```python
from build123d import *

# Parameters (mm, degrees)
SKETCH1_W           = 121.92
SKETCH1_H           = 63.5
BOSS_EXTRUDE1_DEPTH = 5.08
FILLET1_R           = 7.62
SKETCH2_W           = 9.906
SKETCH2_H           = 9.906
BOSS_EXTRUDE2_DEPTH = 22.86
CUT_EXTRUDE2_REACH  = 142.276
SKETCH5_R           = 10.9982
CUT_EXTRUDE3_REACH  = 142.276
SKETCH6_R           = 1.9939
SKETCH7_R           = 5.08
CUT_EXTRUDE4_DEPTH  = 3.81
SKETCH8_R           = 15.24
CUT_EXTRUDE5_DEPTH  = 2.54
CUT_EXTRUDE6_REACH  = 142.276
SKETCH9_R           = 2.159
CUT_EXTRUDE7_REACH  = 142.276
SKETCH11_W          = 143.390320112
SKETCH11_H          = 95.839563071
CUT_EXTRUDE8_DEPTH  = 5.08
SKETCH14_W          = 9.906
SKETCH14_H          = 9.906
BOSS_EXTRUDE4_DEPTH = 7.62
FILLET2_R           = 4.826
FILLET3_R           = 5.08
SKETCH15_R          = 1.27
CUT_EXTRUDE10_DEPTH = 20.32
CUT_EXTRUDE11_REACH = 142.804
SKETCH16_R          = 2.413
CUT_EXTRUDE12_START = -2.54
SKETCH17_W          = 6.096
SKETCH17_H          = 25.146
SKETCH17_W_2        = 2.38136189
SKETCH17_H_2        = 4.064
CUT_EXTRUDE12_DEPTH = 2.54
CUT_EXTRUDE13_REACH = 142.804


with BuildPart() as part:
    # Sketch1 → Boss-Extrude1 (new body)
    with BuildSketch(Plane(origin=(0, 0, 0), x_dir=(1, 0, 0), z_dir=(0, 1, 0))):
        with Locations((60.96, 31.75)):
            Rectangle(SKETCH1_W, SKETCH1_H)
    extrude(amount=BOSS_EXTRUDE1_DEPTH)

    # Fillet1
    fillet1_edges = [part.edges().sort_by_distance(p)[0] for p in [
        (0, 2.54, -63.5),
        (121.92, 2.54, -63.5),
        (121.92, 2.54, 0),
        (0, 2.54, 0),
    ]]
    fillet(fillet1_edges, radius=FILLET1_R)

    # Sketch2 → Boss-Extrude2 (add)
    with BuildSketch(Plane(origin=(0, 5.08, 0), x_dir=(1, 0, 0), z_dir=(0, 1, 0))):
        with Locations((7.747, 55.753)):
            Rectangle(SKETCH2_W, SKETCH2_H)
        with Locations((114.173, 55.753)):
            Rectangle(SKETCH2_W, SKETCH2_H)
        with Locations((114.173, 7.747)):
            Rectangle(SKETCH2_W, SKETCH2_H)
        with Locations((7.747, 7.747)):
            Rectangle(SKETCH2_W, SKETCH2_H)
    extrude(amount=BOSS_EXTRUDE2_DEPTH)

    # Sketch5 → Cut-Extrude2 (cut, up to next)
    with BuildSketch(Plane.XZ, mode=Mode.PRIVATE) as cut_extrude2_sk1:
        with Locations(Location((49.276, -31.75, 0), (0, 0, 270))):
            Circle(SKETCH5_R)
    cut_extrude2_tool1 = extrude(cut_extrude2_sk1.sketch, amount=-CUT_EXTRUDE2_REACH, mode=Mode.PRIVATE) & part.part
    add(cut_extrude2_tool1.solids().sort_by_distance((49.276, 0, -31.75))[0], mode=Mode.SUBTRACT)

    # Sketch6 → Cut-Extrude3 (cut, up to next)
    with BuildSketch(Plane.XZ, mode=Mode.PRIVATE) as cut_extrude3_sk1:
        with Locations(Location((25.4, -16.51, 0), (0, 0, 270))):
            Circle(SKETCH6_R)
    cut_extrude3_tool1 = extrude(cut_extrude3_sk1.sketch, amount=-CUT_EXTRUDE3_REACH, mode=Mode.PRIVATE) & part.part
    # Sketch6 → Cut-Extrude3 (cut, up to next)
    with BuildSketch(Plane.XZ, mode=Mode.PRIVATE) as cut_extrude3_sk2:
        with Locations(Location((25.4, -46.99, 0), (0, 0, 270))):
            Circle(SKETCH6_R)
    cut_extrude3_tool2 = extrude(cut_extrude3_sk2.sketch, amount=-CUT_EXTRUDE3_REACH, mode=Mode.PRIVATE) & part.part
    add(cut_extrude3_tool1.solids().sort_by_distance((25.4, 0, -16.51))[0], mode=Mode.SUBTRACT)
    add(cut_extrude3_tool2.solids().sort_by_distance((25.4, 0, -46.99))[0], mode=Mode.SUBTRACT)

    # Sketch7 → Cut-Extrude4 (cut)
    with BuildSketch(Plane(origin=(0, 5.08, 0), x_dir=(1, 0, 0), z_dir=(0, 1, 0))):
        with Locations(Location((25.4, 46.99, 0), (0, 0, 270))):
            Circle(SKETCH7_R)
        with Locations(Location((25.4, 16.51, 0), (0, 0, 270))):
            Circle(SKETCH7_R)
    extrude(amount=-CUT_EXTRUDE4_DEPTH, mode=Mode.SUBTRACT)

    # Sketch8 → Cut-Extrude5 (cut)
    with BuildSketch(Plane(origin=(0, 5.08, 0), x_dir=(1, 0, 0), z_dir=(0, 1, 0))):
        with Locations(Location((49.276, 31.75, 0), (0, 0, 270))):
            Circle(SKETCH8_R)
    extrude(amount=-CUT_EXTRUDE5_DEPTH, mode=Mode.SUBTRACT)

    # Sketch9 → Cut-Extrude6 (cut, up to next)
    with BuildSketch(Plane.XZ, mode=Mode.PRIVATE) as cut_extrude6_sk1:
        with Locations(Location((25.4, -16.51, 0), (0, 0, 270))):
            Circle(SKETCH9_R)
    cut_extrude6_tool1 = extrude(cut_extrude6_sk1.sketch, amount=-CUT_EXTRUDE6_REACH, mode=Mode.PRIVATE) & part.part
    # Sketch9 → Cut-Extrude6 (cut, up to next)
    with BuildSketch(Plane.XZ, mode=Mode.PRIVATE) as cut_extrude6_sk2:
        with Locations(Location((25.4, -46.99, 0), (0, 0, 270))):
            Circle(SKETCH9_R)
    cut_extrude6_tool2 = extrude(cut_extrude6_sk2.sketch, amount=-CUT_EXTRUDE6_REACH, mode=Mode.PRIVATE) & part.part
    add(cut_extrude6_tool1.solids().sort_by_distance((25.4, 0, -16.51))[0], mode=Mode.SUBTRACT)
    add(cut_extrude6_tool2.solids().sort_by_distance((25.4, 0, -46.99))[0], mode=Mode.SUBTRACT)

    # Sketch10 → Cut-Extrude7 (cut, up to next)
    with BuildSketch(Plane.XZ, mode=Mode.PRIVATE) as cut_extrude7_sk1:
        with BuildLine():
            Line((52.324, -42.502333328), (52.324, -43.561))
            Line((52.324, -43.561), (46.228, -43.561))
            Line((46.228, -43.561), (46.228, -42.502333328))
            ThreePointArc((46.228, -42.502333328), (40.758626429, -38.985836057), (38.172393559, -33.02))
            Line((38.172393559, -33.02), (36.957, -33.02))
            Line((36.957, -33.02), (36.957, -30.48))
            Line((36.957, -30.48), (38.172393559, -30.48))
            ThreePointArc((38.172393559, -30.48), (40.758626429, -24.514163943), (46.228, -20.997666672))
            Line((46.228, -20.997666672), (46.228, -19.939))
            Line((46.228, -19.939), (52.324, -19.939))
            Line((52.324, -19.939), (52.324, -20.997666672))
            ThreePointArc((52.324, -20.997666672), (60.452, -31.75), (52.324, -42.502333328))
        make_face()
    cut_extrude7_tool1 = extrude(cut_extrude7_sk1.sketch, amount=-CUT_EXTRUDE7_REACH, mode=Mode.PRIVATE) & part.part
    add(cut_extrude7_tool1.solids().sort_by_distance((49.190062, 0, -31.75))[0], mode=Mode.SUBTRACT)

    # Sketch11 → Cut-Extrude8 (cut)
    with BuildSketch(Plane(origin=(0, 27.94, 0), x_dir=(1, 0, 0), z_dir=(0, 1, 0))):
        with Locations((59.888985007, 35.781035454)):
            Rectangle(SKETCH11_W, SKETCH11_H)
    extrude(amount=-CUT_EXTRUDE8_DEPTH, mode=Mode.SUBTRACT)

    # Sketch14 → Boss-Extrude4 (add)
    with BuildSketch(Plane(origin=(0, 22.86, 0), x_dir=(1, 0, 0), z_dir=(0, 1, 0))):
        with Locations((114.173, 7.747)):
            Rectangle(SKETCH14_W, SKETCH14_H)
        with Locations((7.747, 7.747)):
            Rectangle(SKETCH14_W, SKETCH14_H)
        with Locations((114.173, 55.753)):
            Rectangle(SKETCH14_W, SKETCH14_H)
        with Locations((7.747, 55.753)):
            Rectangle(SKETCH14_W, SKETCH14_H)
    extrude(amount=BOSS_EXTRUDE4_DEPTH)

    # Fillet2
    fillet2_edges = [part.edges().sort_by_distance(p)[0] for p in [
        (2.794, 17.78, -2.794),
        (119.126, 17.78, -2.794),
        (119.126, 17.78, -60.706),
        (2.794, 17.78, -60.706),
    ]]
    fillet(fillet2_edges, radius=FILLET2_R)

    # Fillet3
    fillet3_edges = [part.edges().sort_by_distance(p)[0] for p in [
        (12.7, 17.78, -12.7),
        (109.22, 17.78, -12.7),
        (109.22, 17.78, -50.8),
        (12.7, 17.78, -50.8),
    ]]
    fillet(fillet3_edges, radius=FILLET3_R)

    # Sketch15 → Cut-Extrude10 (cut)
    with BuildSketch(Plane(origin=(0, 30.48, 0), x_dir=(1, 0, 0), z_dir=(0, 1, 0))):
        with Locations(Location((114.3, 7.62, 0), (0, 0, 270))):
            Circle(SKETCH15_R)
        with Locations(Location((7.62, 7.62, 0), (0, 0, 270))):
            Circle(SKETCH15_R)
        with Locations(Location((114.3, 55.88, 0), (0, 0, 270))):
            Circle(SKETCH15_R)
        with Locations(Location((7.62, 55.88, 0), (0, 0, 270))):
            Circle(SKETCH15_R)
    extrude(amount=-CUT_EXTRUDE10_DEPTH, mode=Mode.SUBTRACT)

    # Sketch16 → Cut-Extrude11 (cut, up to next)
    with BuildSketch(Plane.XZ, mode=Mode.PRIVATE) as cut_extrude11_sk1:
        with Locations(Location((25.4, -16.51, 0), (0, 0, 270))):
            Circle(SKETCH16_R)
    cut_extrude11_tool1 = extrude(cut_extrude11_sk1.sketch, amount=-CUT_EXTRUDE11_REACH, mode=Mode.PRIVATE) & part.part
    # Sketch16 → Cut-Extrude11 (cut, up to next)
    with BuildSketch(Plane.XZ, mode=Mode.PRIVATE) as cut_extrude11_sk2:
        with Locations(Location((25.4, -46.99, 0), (0, 0, 270))):
            Circle(SKETCH16_R)
    cut_extrude11_tool2 = extrude(cut_extrude11_sk2.sketch, amount=-CUT_EXTRUDE11_REACH, mode=Mode.PRIVATE) & part.part
    add(cut_extrude11_tool1.solids().sort_by_distance((25.4, 0, -16.51))[0], mode=Mode.SUBTRACT)
    add(cut_extrude11_tool2.solids().sort_by_distance((25.4, 0, -46.99))[0], mode=Mode.SUBTRACT)

    # Sketch17 → Cut-Extrude12 (cut)
    with BuildSketch(Plane.XZ.offset(CUT_EXTRUDE12_START)):
        with Locations((49.276, -31.75)):
            Rectangle(SKETCH17_W, SKETCH17_H)
        with Locations((37.385680945, -31.75)):
            Rectangle(SKETCH17_W_2, SKETCH17_H_2)
    extrude(amount=CUT_EXTRUDE12_DEPTH, mode=Mode.SUBTRACT)

    # Sketch18 → Cut-Extrude13 (cut, up to next)
    with BuildSketch(Plane.XZ, mode=Mode.PRIVATE) as cut_extrude13_sk1:
        with BuildLine():
            Line((106.68, -13.97), (101.6, -13.97))
            ThreePointArc((101.6, -13.97), (97.79, -10.16), (101.6, -6.35))
            Line((101.6, -6.35), (106.68, -6.35))
            ThreePointArc((106.68, -6.35), (110.49, -10.16), (106.68, -13.97))
        make_face()
    cut_extrude13_tool1 = extrude(cut_extrude13_sk1.sketch, amount=-CUT_EXTRUDE13_REACH, mode=Mode.PRIVATE) & part.part
    # Sketch18 → Cut-Extrude13 (cut, up to next)
    with BuildSketch(Plane.XZ, mode=Mode.PRIVATE) as cut_extrude13_sk2:
        with BuildLine():
            Line((88.9, -13.97), (83.82, -13.97))
            ThreePointArc((83.82, -13.97), (80.01, -10.16), (83.82, -6.35))
            Line((83.82, -6.35), (88.9, -6.35))
            ThreePointArc((88.9, -6.35), (92.71, -10.16), (88.9, -13.97))
        make_face()
    cut_extrude13_tool2 = extrude(cut_extrude13_sk2.sketch, amount=-CUT_EXTRUDE13_REACH, mode=Mode.PRIVATE) & part.part
    # Sketch18 → Cut-Extrude13 (cut, up to next)
    with BuildSketch(Plane.XZ, mode=Mode.PRIVATE) as cut_extrude13_sk3:
        with BuildLine():
            Line((88.9, -57.15), (83.82, -57.15))
            ThreePointArc((83.82, -57.15), (80.01, -53.34), (83.82, -49.53))
            Line((83.82, -49.53), (88.9, -49.53))
            ThreePointArc((88.9, -49.53), (92.71, -53.34), (88.9, -57.15))
        make_face()
    cut_extrude13_tool3 = extrude(cut_extrude13_sk3.sketch, amount=-CUT_EXTRUDE13_REACH, mode=Mode.PRIVATE) & part.part
    # Sketch18 → Cut-Extrude13 (cut, up to next)
    with BuildSketch(Plane.XZ, mode=Mode.PRIVATE) as cut_extrude13_sk4:
        with BuildLine():
            Line((106.68, -57.15), (101.6, -57.15))
            ThreePointArc((101.6, -57.15), (97.79, -53.34), (101.6, -49.53))
            Line((101.6, -49.53), (106.68, -49.53))
            ThreePointArc((106.68, -49.53), (110.49, -53.34), (106.68, -57.15))
        make_face()
    cut_extrude13_tool4 = extrude(cut_extrude13_sk4.sketch, amount=-CUT_EXTRUDE13_REACH, mode=Mode.PRIVATE) & part.part
    add(cut_extrude13_tool1.solids().sort_by_distance((104.14, 0, -10.16))[0], mode=Mode.SUBTRACT)
    add(cut_extrude13_tool2.solids().sort_by_distance((86.36, 0, -10.16))[0], mode=Mode.SUBTRACT)
    add(cut_extrude13_tool3.solids().sort_by_distance((86.36, 0, -53.34))[0], mode=Mode.SUBTRACT)
    add(cut_extrude13_tool4.solids().sort_by_distance((104.14, 0, -53.34))[0], mode=Mode.SUBTRACT)


solid = part.part
```
Here's how the part is built. I have some questions about the finished solid (model axes, mm). A direction names the side the tool comes from. Round coordinates to 2 decimals unless told otherwise and drop trailing zeros. Order: outer loops, then holes, each group sorted by start corner. A loop starts at its lowest first (then second) coordinate and runs counter-clockwise, first axis right, second up. Notation, with made-up numbers: M 70.5,-27 L 88.5,-27 A22 cw 88.5,-16 Z; hole C 33,-38.5 d8. An arc over 180 degrees is marked long. Answer in a Markdown table with one row per item.
Item 1: I'm going to push flat-ended pins straight in: pin 1 (1.4 mm diameter, centred on y = 18.5, z = -59, fed in from -X); pin 2 (1.5 mm diameter, centred on y = 7.5, z = -8, fed in from -X); pin 3 (2.5 mm diameter, centred on y = 16, z = -58.5, fed in from +X). Where does each tip first touch, or does it pass through?
A:
| item | result |
|---|---|
| pin 1 | stops at x = 3.44 |
| pin 2 | stops at x = 2.79 |
| pin 3 | stops at x = 118.93 |
Item 2: If I drill on L1, parallel to Z at x = 25, y = 3; L2, parallel to X at y = 2, z = -53.5; L3, parallel to Z at x = 24, y = 2, over which ranges is the centre line in solid material (lowest first)? Write a range as from..to.
A:
| item | result |
|---|---|
| L1 | z = -63.5..-52.05, -41.93..-21.57, -11.45..0 |
| L2 | x = 0..80.01, 92.71..97.79, 110.49..121.92 |
| L3 | z = -63.5..-51.87, -42.11..-21.39, -11.63..0 |
Item 3: For faces 4 (the face through (109.22, 18, -5)), 5 (the face through (24, 1.27, -14)), 6 (the face through (2.794, 18, -53)), which set-ups out of +Z, -Z, +X, -X, +Y, -Y let a thin tool reach every point of the face, with its end or its side?
A:
| item | result |
|---|---|
| face 4 | +Z, -Z, +Y |
| face 5 | +Y |
| face 6 | +Z, -Z, -X, +Y |
Item 4: Imagine slicing it at C-C, the plane z = -31.75. Write out the boundary of the cut face in (x, y) (3 decimals).
A:
| item | result |
|---|---|
| outline | M 0,0 L 36.195,0 L 36.195,2.54 L 34.036,2.54 L 34.036,5.08 L 0,5.08 Z; M 60.452,0 L 121.92,0 L 121.92,5.08 L 64.516,5.08 L 64.516,2.54 L 60.452,2.54 Z |
Item 5: Imagine slicing it at A-A, the plane y = 20. State how many separate pieces and enclosed holes the cut face has, and give its area (3 significant figures).
A:
| item | result |
|---|---|
| separate pieces | 4 |
| enclosed holes | 4 |
| area | 326 mm2 |
Item 6: Imagine slicing it at D-D, the plane z = -23. Write out the boundary of the cut face in (x, y), and give its area (3 significant figures).
A:
| item | result |
|---|---|
| outline | M 0,0 L 42.32,0 L 42.32,2.54 L 36.8,2.54 L 36.8,5.08 L 0,5.08 Z; M 56.23,0 L 121.92,0 L 121.92,5.08 L 61.75,5.08 L 61.75,2.54 L 56.23,2.54 Z |
| area | 521 mm2 |
Item 7: Imagine slicing it at B-B, the plane x = 25.4. Write out the boundary of the cut face in (y, z).
A:
| item | result |
|---|---|
| outline | M 0,-63.5 L 5.08,-63.5 L 5.08,-52.07 L 1.27,-52.07 L 1.27,-49.4 L 0,-49.4 Z; M 0,-44.58 L 1.27,-44.58 L 1.27,-41.91 L 5.08,-41.91 L 5.08,-21.59 L 1.27,-21.59 L 1.27,-18.92 L 0,-18.92 Z; M 0,-14.1 L 1.27,-14.1 L 1.27,-11.43 L 5.08,-11.43 L 5.08,0 L 0,0 Z |
Item 8: Thinking about a two-plate mould opening in X: for faces 1 (the face through (119.126, 18, -10)), 2 (the face through (10, 18, -2.794)), 3 (the face through (12.7, 18, -58)), which applies, +X half, -X half, draft (parallel to the pull), parting line (faces both ways), or undercut?
A:
| item | result |
|---|---|
| face 1 | +X half |
| face 2 | draft |
| face 3 | undercut |
